Work out the finished part from the listing and answer in its coordinate system (mm). A direction names the side the tool comes from. Coordinates: 2 decimals unless noted, no trailing zeros. Write each loop counter-clockwise with the first axis right and the second up, starting at its lowest first coordinate (ties: lowest second). Pieces come first, ordered by that corner, then holes. Notation, with made-up numbers: M 53.5,84.5 L 66.5,84.5 A17 cw 66.5,97.5 Z; hole C -37.75,35 d10. An arc over 180 degrees is marked long. Answer as CSV lines item,"result". Start each with the question number.
(1) Find the intervals of material crossed by L1, parallel to Y at x = -29.5, z = 3.25; L2, parallel to X at y = 0.25, z = 2; L3, parallel to X at y = -3.5, z = 4.25, in increasing order. Write a range as [from, to].
(2) A cutting plane is placed at D-D on z = 2.5. Count the separate pieces of the cut face and the enclosed holes in it, then the cut area to 3 significant figures.
(3) The mould has two halves that part along Y. Classify faces 3 (the flat face through (0, 3, 12.7)), 4 (the flat face through (2, 1.2, 5.08)), 5 (the flat face through (0, -6.35, 6)): released by +Y, released by -Y, zero draft, split by the parting line, or undercut.
(4) A cutting plane is placed at C-C on y = -4.5. Give the vertices of the cut face in (x, z) (3 decimals).
(5) Flat-ended cylindrical pins translate along their axes: P1, Ø7.5, axis at x = -29.845, y = -0.889, coming from the -Z side; P2, Ø3, axis at x = 29, y = -0.5, coming from the -Z side. Find the tip coordinate at first contact, or state that the pin passes through.
(6) A cutting plane is placed at A-A on x = 0. Give the vertices of the cut face in (y, z).
(7) A cutting plane is placed at B-B on z = 8.89. Give the vertices of the cut face in (x, y) (3 decimals), then the cut area to 3 significant figures.
(8) For faces 1 (the flat face through (32, 1, 5.08)), 2 (the flat face through (0, 6.35, 6)), determine the directions among +Z, -Z, +X, -X, +Y, -Y from which every point of the face is accessible in a straight line to the end or side of a thin tool.
Autodesk Inventor part; units mm, degrees
ref_plane "YZ Plane" through (0, 0, 0) normal (1, 0, 0) x (0, 1, 0)
ref_plane "XZ Plane" through (0, 0, 0) normal (0, 1, 0) x (-1, 0, 0)
ref_plane "XY Plane" through (0, 0, 0) normal (0, 0, 1) x (1, 0, 0)
sketch "Sketch1" plane through (0, 0, 0) normal (0, 0, 1) x (1, 0, 0)
  line L0 (35.56, -6.35) -> (-35.56, -6.35)
  line L1 (-35.56, -6.35) -> (-35.56, 6.35)
  line L2 (-35.56, 6.35) -> (35.56, 6.35)
  line L3 (35.56, 6.35) -> (35.56, -6.35)
  line L4 (35.56, -6.35) -> (-35.56, 6.35) construction
  line L5 (-35.56, -6.35) -> (35.56, 6.35) construction
  line L6 (0, 8.89) -> (0, -8.89)
  line L7 (-49.784, 0) -> (49.784, 0)
  point P0 (0, 0)
  point P1 (-29.845, -0.889)
  point P2 (0, -0.889)
  point P3 (29.845, -0.889)
  point P4 (0, 0)
  dimension "d0" = 71.12
  dimension "d1" = 12.7
  dimension "d4" = 29.845
  dimension "d5" = 5.461
  dimension "d6" = 29.845
extrude "Extrusion1" add sketch "Sketch1" along normal blind 12.7
hole "Hole1" at (-29.845, -0.889, 0) at (0, -0.889, 0) at (29.845, -0.889, 0) direction (0, 0, 1) diameter 5.2578 end through all counterbore diameter 9.525 counterbore depth 5.08
sketch "Sketch2" plane through (0, 0, 0) normal (1, 0, 0) x (0, 1, 0)
  line L0 (-6.35, 0) -> (-6.35, 12.7)
  line L1 (-6.35, 12.7) -> (6.35, 12.7)
  line L2 (-6.35, 12.7) -> (-7.112, 12.7)
  line L3 (-7.112, 12.7) -> (-7.112, 13.462)
  line L4 (-7.112, 13.462) -> (-6.35, 13.462)
  line L5 (-6.35, 13.462) -> (-6.35, 15.24)
  line L6 (-6.35, 15.24) -> (-8.89, 15.24)
  line L7 (-8.89, 15.24) -> (-8.89, 10.795)
  line L8 (-8.89, 10.795) -> (-6.35, 8.255)
  line L9 (-6.35, 8.255) -> (-6.35, 12.7)
  point P0 (0, 0)
  dimension "d15" = 0.762
  dimension "d16" = 0.762
  dimension "d17" = 2.54
  dimension "d18" = 2.54
  dimension "d19" = 45
  dimension "d20" = 4.445
extrude "Extrusion2" [suppressed]
sketch "Sketch3" plane through (-35.56, -6.35, 0) normal (0, -1, 0) x (1, 0, 0)
  line L0 (35.56, 15.24) -> (35.56, -2.54)
  line L1 (-14.224, 0) -> (85.344, 0)
  point P0 (35.56, 0)
  point P1 (26.035, 5.08)
  point P2 (45.085, 5.08)
  point P3 (10.16, 8.89)
  point P4 (60.96, 8.89)
  dimension "d23" = 9.525
  dimension "d24" = 9.525
  dimension "d35" = 8.89
  dimension "d36" = 8.89
  dimension "d37" = 5.08
  dimension "d38" = 15.875
  dimension "d39" = 15.875
hole "Hole2" at (25.4, -6.35, 8.89) at (9.525, -6.35, 5.08) at (-9.525, -6.35, 5.08) at (-25.4, -6.35, 8.89) direction (0, 1, 0) diameter 2.4638 end through all
fillet "Fillet1" radius 3.175 2 edges at (35.56, 6.35, 6.35) (-35.56, 6.35, 6.35)
properties part number "J005362" material "ALUMINUM, 6061-T651"
Here are the results:
1,L1,"y = [-6.35, -5.64], [3.86, 6.35]"
1,L2,"x = [-35.56, -34.47], [-25.22, -4.62], [4.62, 25.22], [34.47, 35.56]"
1,L3,"x = [-35.56, -33.83], [-25.86, -10.44], [-8.61, -3.98], [3.98, 8.61], [10.44, 25.86], [33.83, 35.56]"
2,separate pieces,"1"
2,enclosed holes,"3"
2,area,"685 mm^2"
3,face 3,"zero draft"
3,face 4,"undercut"
3,face 5,"released by -Y"
4,outline,"M -35.56,0 L -32.95,0 L -32.95,5.08 L -26.74,5.08 L -26.74,0 L -3.105,0 L -3.105,5.08 L 3.105,5.08 L 3.105,0 L 26.74,0 L 26.74,5.08 L 32.95,5.08 L 32.95,0 L 35.56,0 L 35.56,12.7 L -35.56,12.7 Z; hole C -25.4,8.89 d2.464; hole C -9.525,5.08 d2.464; hole C 9.525,5.08 d2.464; hole C 25.4,8.89 d2.464"
5,P1,"stops at z = 5.08"
5,P2,"passes through"
6,outline,"M -6.35,0 L -5.65,0 L -5.65,5.08 L -3.52,5.08 L -3.52,12.7 L -6.35,12.7 Z; M 1.74,5.08 L 3.87,5.08 L 3.87,0 L 6.35,0 L 6.35,12.7 L 1.74,12.7 Z"
7,outline,"M -35.56,-6.35 L -26.632,-6.35 L -26.632,6.35 L -32.385,6.35 A3.175 ccw -35.56,3.175 Z; M -24.168,-6.35 L 24.168,-6.35 L 24.168,6.35 L -24.168,6.35 Z; M 26.632,-6.35 L 35.56,-6.35 L 35.56,3.175 A3.175 ccw 32.385,6.35 L 26.632,6.35 Z; hole C -29.845,-0.889 d5.258; hole C 0,-0.889 d5.258; hole C 29.845,-0.889 d5.258"
7,area,"771 mm^2"
8,face 1,"-Z"
8,face 2,"+Z, -Z, +X, -X, +Y"
